from build123d import *

# Parameters (mm, degrees)
SKETCH_1_W      = 9.9
SKETCH_1_H      = 2.8
SKETCH_1_W_2    = 3
SKETCH_1_H_2    = 3.12
EXTRUDE_1_DEPTH = 3
FILLET_1_R      = 1
FILLET_2_R      = 0.5


with BuildPart() as part:
    # Эскиз1 → Бобышка-Вытянуть1 (new body)
    with BuildSketch(Plane(origin=(0, 0, 0), x_dir=(0, 0, -1), z_dir=(1, 0, 0))):
        Polygon((-13.3, -25.94), (-13.3, -29.06), (-10.5, -29.06), (-10.5, -40), (10.5, -40), (10.5, 40), (-10.5, 40), (-10.5, -25.94), align=None)
        with Locations((0, 35.5)):
            Rectangle(SKETCH_1_W, SKETCH_1_H, mode=Mode.SUBTRACT)
        Rectangle(SKETCH_1_W, SKETCH_1_H, mode=Mode.SUBTRACT)
        with Locations((0, -35.5)):
            Rectangle(SKETCH_1_W, SKETCH_1_H, mode=Mode.SUBTRACT)
        with Locations((-12, 27.5)):
            Rectangle(SKETCH_1_W_2, SKETCH_1_H_2)
    extrude(amount=EXTRUDE_1_DEPTH)

    # Скругление1
    fillet_1_edges = [part.edges().sort_by_distance(p)[0] for p in [
        (1.5, 40, 10.5),
        (1.5, -40, 10.5),
    ]]
    fillet(fillet_1_edges, radius=FILLET_1_R)

    # Скругление2
    fillet_2_edges = [part.edges().sort_by_distance(p)[0] for p in [
        (1.5, -25.94, 13.3),
        (1.5, 25.94, 13.5),
        (1.5, 29.06, 13.5),
        (1.5, 40, -10.5),
        (1.5, -40, -10.5),
        (1.5, -29.06, 13.3),
    ]]
    fillet(fillet_2_edges, radius=FILLET_2_R)


solid = part.part
Could you check a few things on this model? Use its own coordinates, in mm. A direction names the side the tool comes from. Give positions to 0.01 mm unless a question says otherwise; leave off trailing zeros. Write each loop counter-clockwise with the first axis right and the second up, starting at its lowest first coordinate (ties: lowest second). Pieces come first, ordered by that corner, then holes. Notation, with made-up numbers: (71, -39) -> (77, -39) arc R24 cw to (77, -4) -> close; hole circle Ø4 at (21, 65). An arc over 180 degrees is marked (long way). Answer as CSV lines item,"result". Start each with the question number.
(1) I'm going to push flat-ended pins straight in: pin 1 Ø1.2 at (x, z) = (2, 12) entering from +Y; pin 2 Ø0.8 at (x, y) = (1.5, 0) entering from +Z; pin 3 Ø2 at (y, z) = (22.5, -7) entering from -X; pin 4 Ø1 at (x, y) = (2, -26.5) entering from +Z. Where does each tip first touch, or does it pass through?
(2) If we section it at A-A, the plane x = 1.95: Give the number of separate pieces and of enclosed holes in the cut face, and give its area (3 significant figures).
(3) Which directions (+Z, -Z, +X, -X, +Y, -Y) give clear straight access to the entire face, cutting with the end or side of a thin tool? Please do faces 4 (the face through (1, -36, 4.95)), 5 (the face through (1, -27, 13.3)), 6 (the face through (1, -25.94, 12)).
(4) If we mould it in two halves opening along Y, with no side actions, what happens to faces 1 (the face through (1, 40, 0)), 2 (the face through (1, 34, 10.5)), 3 (the face through (1, 34.1, 0))? For each: +Y half, -Y half, draft (parallel to the pull), parting line (faces both ways), or undercut.
(5) If we section it at B-B, the plane z = -3.25: Write out the boundary of the cut face in (x, y).
(6) If we section it at C-C, the plane y = -6: Write out the boundary of the cut face in (x, z), and give its area (3 significant figures).
(7) Please list where these lines run through material, in increasing order: line 1 (Y direction, x = 2.3, z = -1.25); line 2 (Y direction, x = 1.4, z = 12.75); line 3 (Z direction, x = 0.8, y = 36).
Answer list:
1,pin 1,"y = 29.06"
1,pin 2,"z = 10.5"
1,pin 3,"x = 0"
1,pin 4,"z = 13.3"
2,separate pieces,"1"
2,enclosed holes,"3"
2,area,"1,610 mm^2"
3,face 4,"+X, -X"
3,face 5,"+Z, +X, -X, -Y"
3,face 6,"+Z, +X, -X"
4,face 1,"+Y half"
4,face 2,"draft"
4,face 3,"undercut"
5,outline,"(0, -40) -> (3, -40) -> (3, -36.9) -> (0, -36.9) -> close; (0, -34.1) -> (3, -34.1) -> (3, -1.4) -> (0, -1.4) -> close; (0, 1.4) -> (3, 1.4) -> (3, 34.1) -> (0, 34.1) -> close; (0, 36.9) -> (3, 36.9) -> (3, 40) -> (0, 40) -> close"
6,outline,"(0, -10.5) -> (3, -10.5) -> (3, 10.5) -> (0, 10.5) -> close"
6,area,"63.0 mm^2"
7,line 1,"-40 to -36.9, -34.1 to -1.4, 1.4 to 34.1, 36.9 to 40"
7,line 2,"-29.06 to -25.94, 25.94 to 29.06"
7,line 3,"-10.5 to -4.95, 4.95 to 10.5"
